Could you check a few things on this drawing? It's one solid part, dimensions in mm from its lowest x, y, z. A direction names the side the tool comes from. Give positions to 0.01 mm unless a question says otherwise; leave off trailing zeros. Loops run counter-clockwise (first coordinate to the right, second up) from the corner with the lowest first, then second, coordinate; pieces in that order, holes last. Notation, with made-up numbers: M 83.5,50.5 L 100.5,50.5 A19 cw 100.5,87.5 Z; hole C -36,48.5 d8. An arc over 180 degrees is marked long. One line per item, written item: value. Start each with the question number.
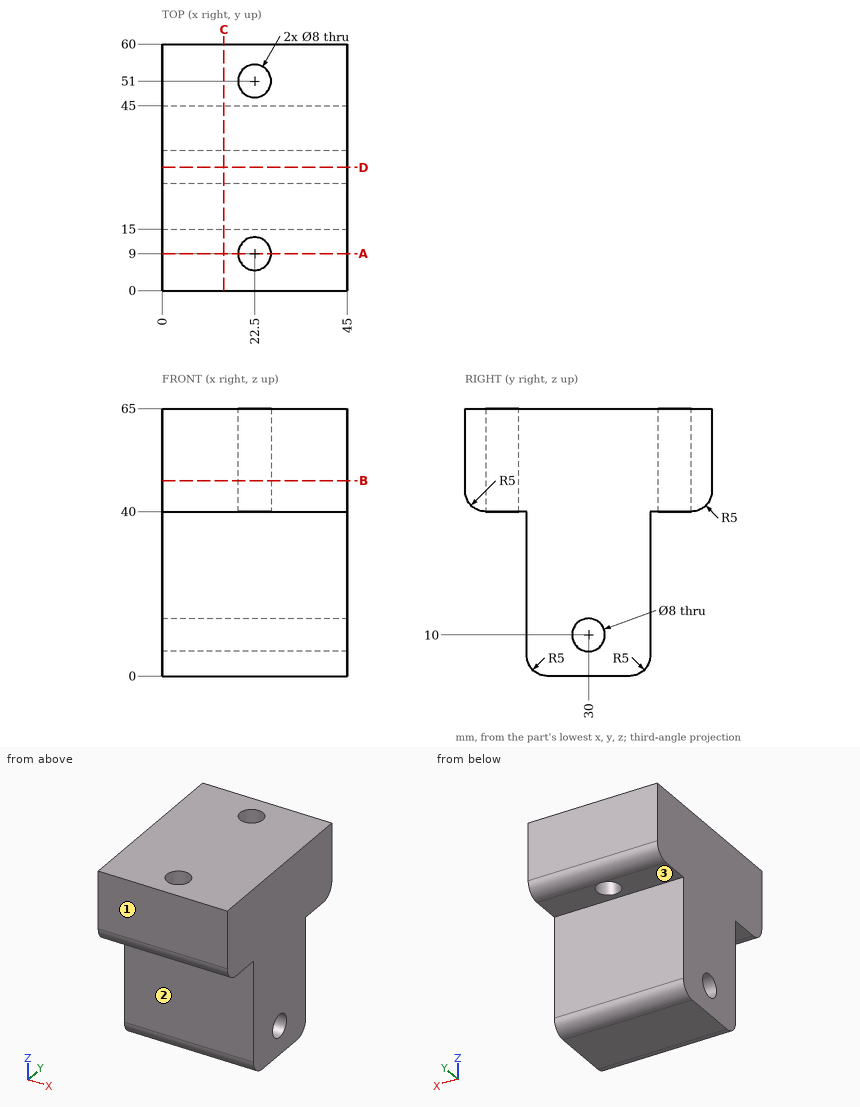
Q1. I need wall thicknesses on line 1 along Z through (x, y) = (35, 30); line 2 along Y through (x, z) = (34.5, 10); line 3 along X through (y, z) = (51, 48.5). Which ranges of each line are inside material? Lowest first, please.
Q2. If we section it at B-B, the plane z = 47.5: Write out the boundary of the cut face in (x, y), plus the area to 3 significant figures.
Q3. If we section it at D-D, the plane y = 30: Write out the boundary of the cut face in (x, z).
Q4. If we section it at C-C, the plane x = 15: Write out the boundary of the cut face in (y, z), plus the area to 3 significant figures.
Q5. If we section it at A-A, the plane y = 9: Write out the boundary of the cut face in (x, z), plus the area to 3 significant figures.
Q6. For P1, Ø10.5, axis at x = 33, z = 24.5, coming from the -Y side; P2, Ø10.5, axis at x = 22.5, y = 9, coming from the +Z side; P3, Ø5, axis at y = 30, z = 10, coming from the -X side; P4, Ø11, axis at x = 32.5, y = 49.5, coming from the -Z side, each with a flat end and sliding along its axis, tell me the tip position at first contact or that it passes through.
Q7. Which directions (+Z, -Z, +X, -X, +Y, -Y) give clear straight access to the entire face, cutting with the end or side of a thin tool? Please do the marked faces 1, 2 and 3.
Response:
1. line 1: 0 to 6, 14 to 65
1. line 2: 15 to 26, 34 to 45
1. line 3: 0 to 18.5, 26.5 to 45
2. outline: M 0,0 L 45,0 L 45,60 L 0,60 Z; hole C 22.5,9 d8; hole C 22.5,51 d8
2. area: 2,600 mm^2
3. outline: M 0,0 L 45,0 L 45,6 L 0,6 Z; M 0,14 L 45,14 L 45,65 L 0,65 Z
4. outline: M 0,45 A5 ccw 5,40 L 15,40 L 15,5 A5 ccw 20,0 L 40,0 A5 ccw 45,5 L 45,40 L 55,40 A5 ccw 60,45 L 60,65 L 0,65 Z; hole C 30,10 d8
4. area: 2,630 mm^2
5. outline: M 0,40 L 18.5,40 L 18.5,65 L 0,65 Z; M 26.5,40 L 45,40 L 45,65 L 26.5,65 Z
5. area: 925 mm^2
6. P1: y = 15
6. P2: z = 65
6. P3: through
6. P4: z = 2
7. face 1: +Z, -Z, +X, -X, -Y
7. face 2: -Z, +X, -X, -Y
7. face 3: -Z, +X, -X, +Y
